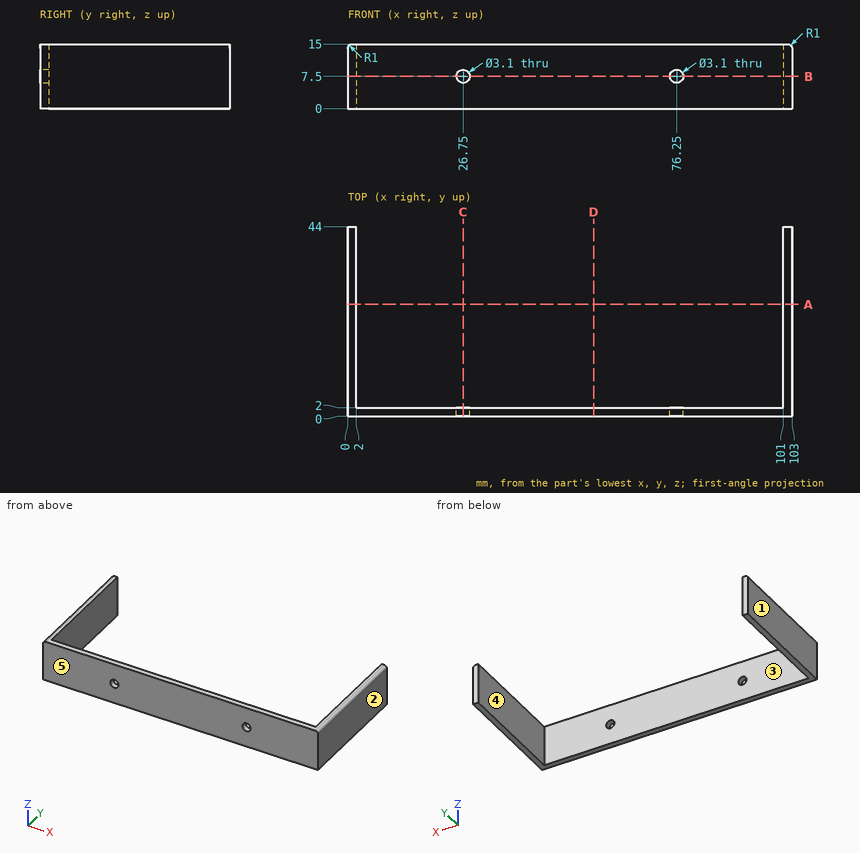
Input: dimensioned drawing with shaded views. Units: mm. Origin: part minimum x, y, z. A direction names the side the tool comes from. Give positions to 0.01 mm unless a question says otherwise; leave off trailing zeros. Loops run counter-clockwise (first coordinate to the right, second up) from the corner with the lowest first, then second, coordinate; pieces in that order, holes last. Notation, with made-up numbers: M 6.5,-21 L 11.5,-21 A20 cw 11.5,-14 Z; hole C 23,-2 d1. An arc over 180 degrees is marked long. Put each result on its own line as item: value. Start each with the question number.
1) Cut plane A-A (y = 26). Output: boundary loops of the cut face in (x, z), then the cut area to 3 significant figures.
2) Cut plane C-C (x = 26.75). Output: boundary loops of the cut face in (y, z).
3) Cut plane D-D (x = 57). Output: boundary loops of the cut face in (y, z), then the cut area to 3 significant figures.
4) Access query for the marked faces 4 and 5. Directions: +Z, -Z, +X, -X, +Y, -Y. A direction counts if a zero-diameter tool reaches every point of the face in a straight line with its end or side. Return the directions, or none.
5) Pull-direction query (X, two-part tool) for the marked faces 1, 2 and 3; classes: pulls with the +X half, pulls with the -X half, needs draft (parallel to the pull), parting line crosses it, or undercut.
6) Ray query, line 1 along X through (y, z) = (1.45, 7.5); line 2 along X through (y, z) = (35.5, 8.5); line 3 along Y through (x, z) = (91, 3.75). Return the intervals inside material, ascending.
7) Cut plane B-B (z = 7.5). Output: boundary loops of the cut face in (x, y).
Verdict:
1. outline: M 0,0 L 2,0 L 2,15 L 1,15 A1 ccw 0,14 Z; M 101,0 L 103,0 L 103,14 A1 ccw 102,15 L 101,15 Z
1. area: 59.6 mm2
2. outline: M 0,0 L 2,0 L 2,5.95 L 0,5.95 Z; M 0,9.05 L 2,9.05 L 2,15 L 0,15 Z
3. outline: M 0,0 L 2,0 L 2,15 L 0,15 Z
3. area: 30.0 mm2
4. face 4: +Z, -Z, +Y
4. face 5: +Z, -Z, +X, -X, -Y
5. face 1: pulls with the -X half
5. face 2: pulls with the +X half
5. face 3: undercut
6. line 1: 0 to 25.2, 28.3 to 74.7, 77.8 to 103
6. line 2: 0 to 2, 101 to 103
6. line 3: 0 to 2
7. outline: M 0,0 L 25.2,0 L 25.2,2 L 2,2 L 2,44 L 0,44 Z; M 28.3,0 L 74.7,0 L 74.7,2 L 28.3,2 Z; M 77.8,0 L 103,0 L 103,44 L 101,44 L 101,2 L 77.8,2 Z
